Can you work these out from the model? Positions are in its coordinate system, mm. A direction names the side the tool comes from. Round coordinates to 2 decimals unless told otherwise and drop trailing zeros. Loops run counter-clockwise (first coordinate to the right, second up) from the corner with the lowest first, then second, coordinate; pieces in that order, holes last.
(1) Which directions (+Z, -Z, +X, -X, +Y, -Y) give clear straight access to the entire face, cutting with the end or side of a thin tool? Please do faces 4 (the face through (1, 0, 0)), 5 (the face through (-2.39, 5.12, -4.14)), 6 (the face through (0, 7.62, -5)), 7 (the face through (2.39, 5.12, -4.14)), 8 (the face through (0.023, 5.116, -3.175)).
(2) If I drill on line 1 along Z through (x, y) = (0, 1.45); line 2 along Y through (x, z) = (-4, 0); line 3 along Z through (x, y) = (-3, 5.25), over which ranges is the centre line in solid material (lowest first)?
(3) I want a section at C-C on z = 0. Write out the boundary of the cut face in (x, y), plus the area to 3 significant figures.
(4) Thinking about a two-plate mould opening in Z: for faces 1 (the face through (-1.38, 2.91, 6.2)), 2 (the face through (0, 7.62, 5)), 3 (the face through (-2.37, 5.116, 4.105)), which applies, released by +Z, released by -Z, zero draft, split by the parting line, or undercut?
(5) I want a section at D-D on z = 3.75. Write out the boundary of the cut face in (x, y), plus the area to 3 significant figures.
(6) Will these pins go through, and if not, where does the flat tip stop? pin 1 Ø2 at (x, z) = (-2, -2.5) entering from -Y; pin 2 Ø4 at (x, y) = (2.5, 4.5) entering from +Z; pin 3 Ø1.5 at (x, z) = (-4.5, 5) entering from +Y.
(7) I want a section at A-A on x = 0. Write out the boundary of the cut face in (y, z) (3 decimals).
from build123d import *

# Parameters (mm, degrees)
SKETCH1_R             = 6.35
BOSS_EXTRUDE1_DEPTH   = 7.62
F_0_80_TAPPED_HOLE1_D = 1.19126
SKETCH4_R             = 3.175
CUT_EXTRUDE1_DEPTH    = 5.08
CUT_EXTRUDE2_DEPTH    = 5.08


with BuildPart() as part:
    # Sketch1 → Boss-Extrude1 (new body)
    with BuildSketch(Plane(origin=(0, 0, 0), x_dir=(1, 0, 0), z_dir=(0, 1, 0))):
        Circle(SKETCH1_R)
    extrude(amount=BOSS_EXTRUDE1_DEPTH)

    # #0-80 Tapped Hole1 (through all)
    with Locations(Plane(origin=(0, 7.62, 0), x_dir=(1, 0, 0), z_dir=(0, 1, 0))):
        with Locations((0, 0)):
            Hole(F_0_80_TAPPED_HOLE1_D / 2)

    # Sketch4 → Cut-Extrude1 (cut)
    with BuildSketch(Plane(origin=(0, 7.62, 0), x_dir=(1, 0, 0), z_dir=(0, 1, 0))):
        Circle(SKETCH4_R)
    extrude(amount=-CUT_EXTRUDE1_DEPTH, mode=Mode.SUBTRACT)

    # Sketch5 → Cut-Extrude2 (cut)
    with BuildSketch(Plane(origin=(0, 7.62, 0), x_dir=(1, 0, 0), z_dir=(0, 1, 0))):
        Polygon((0, 0), (-7.62, -13.198227154), (-7.62, 13.198227154), align=None)
    cut_extrude2 = extrude(amount=-CUT_EXTRUDE2_DEPTH, mode=Mode.SUBTRACT)

    # Mirror1: Cut-Extrude2 across plane
    add(cut_extrude2.mirror(Plane(origin=(0, 0, 0), x_dir=(0, 0, 1), z_dir=(1, 0, 0))), mode=Mode.SUBTRACT)


solid = part.part
Filled sheet:
1. face 4: +Z, -Z, +X, -X, -Y
1. face 5: -X, +Y
1. face 6: +Z, -Z, +X, -X, +Y
1. face 7: +X, +Y
1. face 8: +Y
2. line 1: z = -6.35 to -0.6, 0.6 to 6.35
2. line 2: y = 0 to 2.54
2. line 3: z = -5.6 to -5.2, 5.2 to 5.6
3. outline: (-6.35, 0) - (-0.6, 0) - (-0.6, 2.54) - (-6.35, 2.54) - close; (0.6, 0) - (6.35, 0) - (6.35, 2.54) - (0.6, 2.54) - close
3. area: 29.2 mm2
4. face 1: split by the parting line
4. face 2: zero draft
4. face 3: undercut
5. outline: (-5.12, 0) - (5.12, 0) - (5.12, 2.54) - (2.17, 2.54) - (2.17, 7.62) - (-2.17, 7.62) - (-2.17, 2.54) - (-5.12, 2.54) - close
5. area: 48.0 mm2
6. pin 1: stops at y = 0
6. pin 2: stops at z = 6.33
6. pin 3: stops at y = 2.54
7. outline: (0, -6.35) - (7.62, -6.35) - (7.62, -3.175) - (2.54, -3.175) - (2.54, -0.596) - (0, -0.596) - close; (0, 0.596) - (2.54, 0.596) - (2.54, 3.175) - (7.62, 3.175) - (7.62, 6.35) - (0, 6.35) - close
